The drawing under review shows one solid part. Ordinate dimensions are in mm from its lowest x, y, z. A direction names the side the tool comes from. Round coordinates to 2 decimals unless told otherwise and drop trailing zeros. Write each loop counter-clockwise with the first axis right and the second up, starting at its lowest first coordinate (ties: lowest second). Pieces come first, ordered by that corner, then holes. Notation, with made-up numbers: (-1.5, 11.25) -> (43.5, 11.25) arc R17 cw to (43.5, 44.25) -> close; hole circle Ø1 at (35.25, 61). An arc over 180 degrees is marked (long way). Answer in a Markdown table with one row per item.
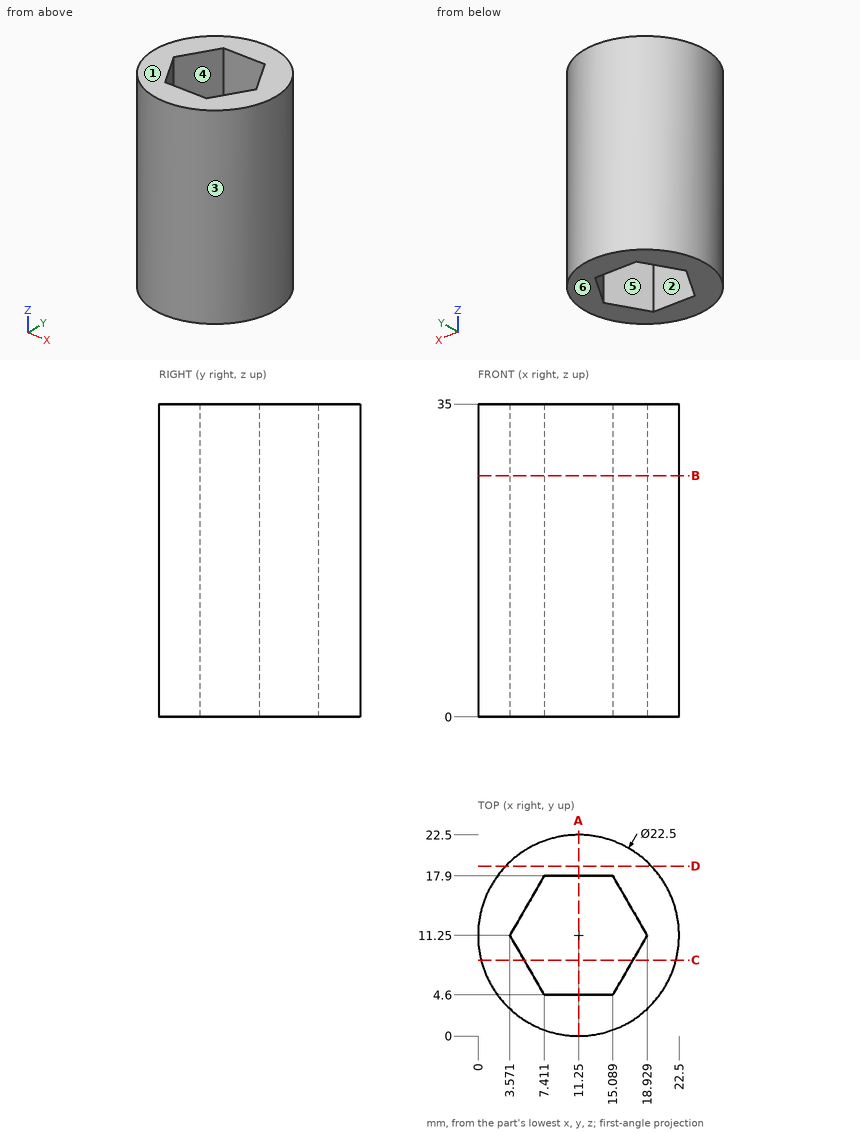
1) For line 1 (Y direction, x = 18.75, z = 29) (1 decimal); line 2 (X direction, y = 10, z = 5.5); line 3 (X direction, y = 14, z = 23), list the stretches that pass through material, from the lowest coordinate up. Write a range as [from, to].
Solved:
| item | result |
|---|---|
| line 1 | [2.9, 10.9], [11.6, 19.6] |
| line 2 | [0.07, 4.29], [18.21, 22.43] |
| line 3 | [0.34, 5.16], [17.34, 22.16] |
2) Clearance check with flat-ended pins moving along their axes: pin 1 Ø2 at (y, z) = (12.5, 13) entering from +X; pin 2 Ø8 at (x, z) = (4, 11.5) entering from +Y; pin 3 Ø6 at (y, z) = (15, 12.5) entering from -X (1 decimal). State where each tip first meets the part, or that it passes through.
Solved:
| item | result |
|---|---|
| pin 1 | x = 22.5 |
| pin 2 | y = 22.02 |
| pin 3 | x = 0 |
3) Consider section C-C on y = 8.5. State the section outline as (x, z) points.
Solved:
| item | result |
|---|---|
| outline | (0.34, 0) -> (5.16, 0) -> (5.16, 35) -> (0.34, 35) -> close; (17.34, 0) -> (22.16, 0) -> (22.16, 35) -> (17.34, 35) -> close |
4) Consider section A-A on x = 11.25. State the section outline as (y, z) points, then the cut area to 3 significant figures.
Solved:
| item | result |
|---|---|
| outline | (0, 0) -> (4.6, 0) -> (4.6, 35) -> (0, 35) -> close; (17.9, 0) -> (22.5, 0) -> (22.5, 35) -> (17.9, 35) -> close |
| area | 322 mm² |
5) Mouldability with a two-part tool opening along X and no side actions: class the marked faces 1, 2, 3 and 4 as pulls with the +X half, pulls with the -X half, needs draft (parallel to the pull), parting line crosses it, or undercut.
Solved:
| item | result |
|---|---|
| face 1 | needs draft |
| face 2 | undercut |
| face 3 | parting line crosses it |
| face 4 | undercut |
6) Consider section D-D on y = 19. State the section outline as (x, z) points (1 decimal), then the cut area to 3 significant figures.
Solved:
| item | result |
|---|---|
| outline | (3.1, 0) -> (19.4, 0) -> (19.4, 35) -> (3.1, 35) -> close |
| area | 571 mm² |
7) For the marked faces 5 and 6, list the 3-axis set-ups (+Z, -Z, +X, -X, +Y, -Y) from which the entire face can be reached by the end or side of a thin tool; tool diameter is ignored.
Solved:
| item | result |
|---|---|
| face 5 | +Z, -Z |
| face 6 | -Z, +X, -X, +Y, -Y |
8) Consider section B-B on z = 27. State the section outline as (x, y) points.
Solved:
| item | result |
|---|---|
| outline | circle Ø22.5 at (11.25, 11.25); hole (3.57, 11.25) -> (7.41, 4.6) -> (15.09, 4.6) -> (18.93, 11.25) -> (15.09, 17.9) -> (7.41, 17.9) -> close |
